Could you check a few things on this model? Use its own coordinates, in mm. Face numbers are marked on the shaded views. Give positions to 0.01 mm unless a question says otherwise; leave off trailing zeros. Order: outer loops, then holes, each group sorted by start corner. A loop starts at its lowest first (then second) coordinate and runs counter-clockwise, first axis right, second up.
(1) If we mould it in two halves opening along X, with no side actions, what happens to the marked faces 1, 2, 3 and 4? For each: released by +X, released by -X, zero draft, split by the parting line, or undercut.
(2) If I drill on probe 1 along Y at (x, z) = (0, 1.15); probe 2 along Y at (x, z) = (-3, 3.75); probe 3 along Y at (x, z) = (13, 0.35), over which ranges is the centre line in solid material (lowest first)?
(3) Imagine slicing it at A-A, the plane x = 9. Write out the boundary of the cut face in (y, z).
(4) Imagine slicing it at C-C, the plane y = 0. Write out the boundary of the cut face in (x, z), then the cut area to 3 significant figures.
(5) Imagine slicing it at D-D, the plane z = 1.2. Write out the boundary of the cut face in (x, y).
(6) Imagine slicing it at B-B, the plane x = 0. Write out the boundary of the cut face in (y, z), then the cut area to 3 significant figures.
(7) Will this pin go through, and if not, where does the flat tip stop? pin 1 (24 mm diameter, centred on x = 0, y = 0, fed in from +Z).
from build123d import *

# Parameters (mm, degrees)
SKETCH_R   = 4
SKETCH_R_2 = 15
PAD_DEPTH  = 5


with BuildPart() as part:
    # Sketch → Pad (new body)
    with BuildSketch(Plane.XY):
        with BuildLine():
            Line((-15.5, 21.15), (15.5, 21.15))
            ThreePointArc((21.15, 15.5), (19.495153, 19.495153), (15.5, 21.15))
            Line((21.15, 15.5), (21.15, -77.362437))
            ThreePointArc((15.5, -83.012437), (19.495153, -81.35759), (21.15, -77.362437))
            Line((15.5, -83.012437), (-15.5, -83.012437))
            ThreePointArc((-21.15, -77.362437), (-19.495153, -81.35759), (-15.5, -83.012437))
            Line((-21.15, -77.362437), (-21.15, 15.5))
            ThreePointArc((-15.5, 21.15), (-19.495153, 19.495153), (-21.15, 15.5))
        make_face()
        with Locations((0, -76.8)):
            Circle(SKETCH_R, mode=Mode.SUBTRACT)
        Circle(SKETCH_R_2, mode=Mode.SUBTRACT)
        with BuildLine():
            ThreePointArc((-17.2, 12.542002), (-15.5, 10.842002), (-13.8, 12.542002))
            Line((-13.8, 12.542002), (-13.8, 17.562841))
            ThreePointArc((-13.8, 17.562841), (-15.5, 19.262841), (-17.2, 17.562841))
            Line((-17.2, 12.542002), (-17.2, 17.562841))
        make_face(mode=Mode.SUBTRACT)
        with BuildLine():
            ThreePointArc((13.8, 12.542002), (15.5, 10.842002), (17.2, 12.542002))
            Line((17.2, 12.542002), (17.2, 17.562841))
            ThreePointArc((17.2, 17.562841), (15.5, 19.262841), (13.8, 17.562841))
            Line((13.8, 12.542002), (13.8, 17.562841))
        make_face(mode=Mode.SUBTRACT)
        with BuildLine():
            ThreePointArc((-13.8, -13.068467), (-15.5, -11.368467), (-17.2, -13.068467))
            Line((-17.2, -13.068467), (-17.2, -18.089305))
            ThreePointArc((-17.2, -18.089305), (-15.5, -19.789305), (-13.8, -18.089305))
            Line((-13.8, -13.068467), (-13.8, -18.089305))
        make_face(mode=Mode.SUBTRACT)
        with BuildLine():
            ThreePointArc((17.2, -13.068467), (15.5, -11.368467), (13.8, -13.068467))
            Line((13.8, -13.068467), (13.8, -18.089305))
            ThreePointArc((13.8, -18.089305), (15.5, -19.789305), (17.2, -18.089305))
            Line((17.2, -13.068467), (17.2, -18.089305))
        make_face(mode=Mode.SUBTRACT)
    extrude(amount=PAD_DEPTH)


solid = part.part
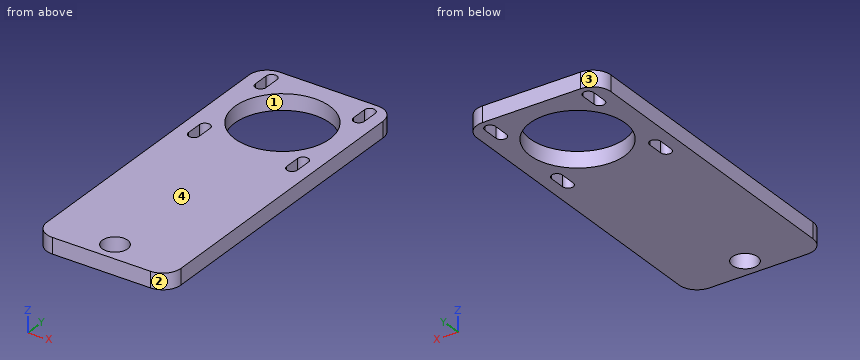
Answer block:
1. face 1: undercut
1. face 2: released by +X
1. face 3: released by -X
1. face 4: zero draft
2. probe 1: y = -83.01 to -80.8, -72.8 to -15, 15 to 21.15
2. probe 2: y = -83.01 to -79.45, -74.15 to -14.7, 14.7 to 21.15
2. probe 3: y = -83.01 to -7.48, 7.48 to 21.15
3. outline: (-83.01, 0) - (-12, 0) - (-12, 5) - (-83.01, 5) - close; (12, 0) - (21.15, 0) - (21.15, 5) - (12, 5) - close
4. outline: (-21.15, 0) - (-15, 0) - (-15, 5) - (-21.15, 5) - close; (15, 0) - (21.15, 0) - (21.15, 5) - (15, 5) - close
4. area: 61.5 mm2
5. outline: (-21.15, -77.36) arc R5.65 ccw to (-15.5, -83.01) - (15.5, -83.01) arc R5.65 ccw to (21.15, -77.36) - (21.15, 15.5) arc R5.65 ccw to (15.5, 21.15) - (-15.5, 21.15) arc R5.65 ccw to (-21.15, 15.5) - close; hole (-17.2, -18.09) arc R1.7 ccw to (-13.8, -18.09) - (-13.8, -13.07) arc R1.7 ccw to (-17.2, -13.07) - close; hole (-17.2, 12.54) arc R1.7 ccw to (-13.8, 12.54) - (-13.8, 17.56) arc R1.7 ccw to (-17.2, 17.56) - close; hole circle Ø30 at (0, 0); hole circle Ø8 at (0, -76.8); hole (13.8, -18.09) arc R1.7 ccw to (17.2, -18.09) - (17.2, -13.07) arc R1.7 ccw to (13.8, -13.07) - close; hole (13.8, 12.54) arc R1.7 ccw to (17.2, 12.54) - (17.2, 17.56) arc R1.7 ccw to (13.8, 17.56) - close
6. outline: (-83.01, 0) - (-80.8, 0) - (-80.8, 5) - (-83.01, 5) - close; (-72.8, 0) - (-15, 0) - (-15, 5) - (-72.8, 5) - close; (15, 0) - (21.15, 0) - (21.15, 5) - (15, 5) - close
6. area: 331 mm2
7. pin 1: passes through
